The model under review builds one solid part; all positions refer to its coordinate system, in mm. Face numbers are marked on the shaded views. Coordinates: 2 decimals unless noted, no trailing zeros. Loops run counter-clockwise (first coordinate to the right, second up) from the corner with the lowest first, then second, coordinate; pieces in that order, holes last. Notation, with made-up numbers: M -11.75,34 L 46.25,34 A14 cw 46.25,60 Z; hole C 24.5,59.5 d1. An arc over 180 degrees is marked long. Use one line per item in the form item = value.
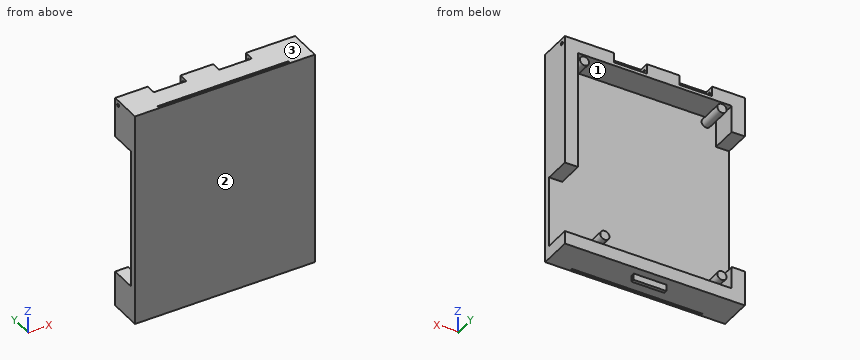
```python
from build123d import *

# Parameters (mm, degrees)
SKETCH1_W           = 47.09
SKETCH1_H           = 58.17
BOSS_EXTRUDE1_DEPTH = 2
SKETCH2_R           = 1.4
BOSS_EXTRUDE2_DEPTH = 8
BOSS_EXTRUDE3_DEPTH = 10
SKETCH6_W           = 4.055357108
SKETCH6_H           = 43.053811849
SKETCH6_W_2         = 4
SKETCH6_H_2         = 21.843851608
CUT_EXTRUDE2_DEPTH  = 8
SKETCH8_R           = 0.5
CUT_EXTRUDE3_DEPTH  = 84.666104248
SKETCH10_R          = 2.134407384
CUT_EXTRUDE4_DEPTH  = 10
SKETCH11_R          = 2.134407384
CUT_EXTRUDE5_DEPTH  = 10
BOSS_EXTRUDE4_DEPTH = 2
SKETCH13_W          = 39.99
SKETCH13_H          = 0.463806664
CUT_EXTRUDE6_DEPTH  = 85.194162505


with BuildPart() as part:
    # Sketch1 → Boss-Extrude1 (new body)
    with BuildSketch(Plane(origin=(0, 0, 0), x_dir=(1, 0, 0), z_dir=(0, 1, 0))):
        with Locations((23.545, -29.085)):
            Rectangle(SKETCH1_W, SKETCH1_H)
    extrude(amount=BOSS_EXTRUDE1_DEPTH)

    # Sketch2 → Boss-Extrude2 (add)
    with BuildSketch(Plane(origin=(0, 2, 0), x_dir=(1, 0, 0), z_dir=(0, 1, 0))):
        with Locations(Location((38.86, -3, 0), (0, 0, 90))):
            Circle(SKETCH2_R)
        with Locations(Location((45.09, -56.32, 0), (0, 0, 90))):
            Circle(SKETCH2_R)
        with Locations(Location((3, -56.32, 0), (0, 0, 90))):
            Circle(SKETCH2_R)
        with Locations(Location((3, -3, 0), (0, 0, 90))):
            Circle(SKETCH2_R)
    extrude(amount=BOSS_EXTRUDE2_DEPTH)

    # Sketch3 → Boss-Extrude3 (add)
    with BuildSketch(Plane(origin=(0, 0, 0), x_dir=(1, 0, 0), z_dir=(0, 1, 0))):
        Polygon((0, -26.469922438), (0, 0), (23.66505447, 0), (23.66505447, 4), (-4, 4), (-4, -26.469922438), align=None)
        Polygon((23.66505447, 4), (23.66505447, 0), (47.09, 0), (47.09, -29.085), (51.09, -29.085), (51.09, 4), align=None)
        Polygon((47.09, -58.17), (23.66505447, -58.17), (23.66505447, -62.17), (51.09, -62.17), (51.09, -29.085), (47.09, -29.085), align=None)
        Polygon((0, -58.17), (0, -26.469922438), (-4, -26.469922438), (-4, -62.17), (23.66505447, -62.17), (23.66505447, -58.17), align=None)
    extrude(amount=BOSS_EXTRUDE3_DEPTH)

    # Sketch6 → Cut-Extrude2 (cut)
    with BuildSketch(Plane(origin=(0, 10, 0), x_dir=(1, 0, 0), z_dir=(0, 1, 0))):
        with Locations((-1.972321446, -28.345718343)):
            Rectangle(SKETCH6_W, SKETCH6_H)
        with Locations((49.09, -10.921925804)):
            Rectangle(SKETCH6_W_2, SKETCH6_H_2)
    extrude(amount=-CUT_EXTRUDE2_DEPTH, mode=Mode.SUBTRACT)

    # Sketch8 → Cut-Extrude3 (cut, through all)
    with BuildSketch(Plane(origin=(51.09, 0, 0), x_dir=(0, 0, -1), z_dir=(1, 0, 0))):
        with Locations((-60.66237095, 8.489122927)):
            Circle(SKETCH8_R)
    extrude(amount=-CUT_EXTRUDE3_DEPTH, mode=Mode.SUBTRACT)

    # Sketch10 → Cut-Extrude4 (cut)
    with BuildSketch(Plane(origin=(6, 10, 62.17), x_dir=(0, 0, -1), z_dir=(1, 0, 0))):
        with Locations((1.50762905, -1.510877073)):
            Circle(SKETCH10_R)
    extrude(amount=CUT_EXTRUDE4_DEPTH, mode=Mode.SUBTRACT)

    # Sketch11 → Cut-Extrude5 (cut)
    with BuildSketch(Plane(origin=(26, 10, 62.17), x_dir=(0, 0, -1), z_dir=(1, 0, 0))):
        with Locations((1.50762905, -1.510877073)):
            Circle(SKETCH11_R)
    extrude(amount=CUT_EXTRUDE5_DEPTH, mode=Mode.SUBTRACT)

    # Sketch12 → Boss-Extrude4 (add)
    with BuildSketch(Plane(origin=(0, 0, -4), x_dir=(-1, 0, 0), z_dir=(0, 0, -1))):
        Polygon((-23.54, 7.513197032), (-28.54, 7.513197032), (-28.54, 6.476270602), (-18.54, 6.476270602), (-18.54, 7.513197032), align=None)
    extrude(amount=BOSS_EXTRUDE4_DEPTH)

    # Sketch13 → Cut-Extrude6 (cut, through all)
    with BuildSketch(Plane(origin=(0, 0, -4), x_dir=(-1, 0, 0), z_dir=(0, 0, -1))):
        with Locations((-23.545, 0.728666672)):
            Rectangle(SKETCH13_W, SKETCH13_H)
    extrude(amount=-CUT_EXTRUDE6_DEPTH, mode=Mode.SUBTRACT)


solid = part.part
```
1. Add section D-D (x = 45.09). State the section outline as (y, z) points.
Response values:
outline = M 0,-4 L 10,-4 L 10,0 L 2,0 L 2,54.92 L 10,54.92 L 10,57.72 L 2,57.72 L 2,58.17 L 10,58.17 L 10,62.17 L 0,62.17 Z; hole C 8.49,60.66 d1
2. Add section C-C (y = 3.25). State the section outline as (x, z) points, then the cut area to 3 significant figures.
Response values:
outline = M -4,-4 L 51.09,-4 L 51.09,0 L 0,0 L 0,6.82 L -4,6.82 Z; M -4,49.87 L 0,49.87 L 0,58.17 L 47.09,58.17 L 47.09,21.84 L 51.09,21.84 L 51.09,62.17 L -4,62.17 Z; C 3,3 d2.8; C 3,56.32 d2.8; C 38.86,3 d2.8; C 45.09,56.32 d2.8
area = 671 mm^2
3. Insertion check: P1, Ø1, axis at x = 22, z = -5, coming from the +Y side; P2, Ø5, axis at x = 45.5, y = 3.5, coming from the -Z side; P3, Ø4, axis at x = 39.5, z = 48, coming from the -Y side; P4, Ø0.5, axis at y = 7, z = -5, coming from the -X side. Each pin has a flat end and moves straight along its axis. Give the tip position at first contact, or say it passes through.
Response values:
P1 = 7.51
P2 = -4
P3 = 0
P4 = 18.54
4. Wall thickness on line 1 along Z through (x, y) = (33.5, 5.5); line 2 along Z through (x, y) = (46, 9.5); line 3 along Y through (x, z) = (32.5, 8): over which ranges is each line inside the solid? List them lowest first. Write a range as from..to.
Response values:
line_1 = -4..0, 58.17..62.17
line_2 = -4..0, 55.26..57.38, 58.17..62.17
line_3 = 0..0.5, 0.96..2
5. Add section A-A (z = -1). State the section outline as (x, y) points.
Response values:
outline = M -4,0 L 51.09,0 L 51.09,10 L -4,10 Z; hole M 3.55,0.5 L 43.54,0.5 L 43.54,0.96 L 3.55,0.96 Z
6. The part is to be moulded in two halves that separate along Z. For the marked faces 1, 2 and 3, say which applies: pulls with the +Z half, pulls with the -Z half, needs draft (parallel to the pull), parting line crosses it, or undercut.
Response values:
face_1 = undercut
face_2 = needs draft
face_3 = pulls with the +Z half
7. Add section B-B (x = 23.5). State the section outline as (y, z) points, then the cut area to 3 significant figures.
Response values:
outline = M 0,-4 L 0.5,-4 L 0.5,62.17 L 0,62.17 Z; M 0.96,-4 L 6.48,-4 L 6.48,-6 L 7.51,-6 L 7.51,-4 L 10,-4 L 10,0 L 2,0 L 2,58.17 L 10,58.17 L 10,62.17 L 0.96,62.17 Z; hole C 8.49,60.66 d1
area = 167 mm^2
